The model under review builds one solid part; all positions refer to its coordinate system, in mm. A direction names the side the tool comes from. Give positions to 0.01 mm unless a question says otherwise; leave off trailing zeros. Loops run counter-clockwise (first coordinate to the right, second up) from the corner with the lowest first, then second, coordinate; pieces in that order, holes last. Notation, with made-up numbers: (14.25, 54) -> (46.25, 54) arc R13 cw to (46.25, 63) -> close; hole circle Ø8 at (-33, -8.5). An arc over 180 degrees is marked (long way). Write each question's results on one line, items separated by ' | '. Start each with the question number.
Q1. Mouldability with a two-part tool opening along X and no side actions: class faces 4 (the face through (-4.166, 1.398, 3.732)), 5 (the face through (11.68, 0.78, 3.7)), 6 (the face through (7, 1, 7.5)) as released by +X, released by -X, zero draft, split by the parting line, or undercut.
Q2. Insertion check: pin 1 Ø1.1 at (x, y) = (0, 0) entering from +Z; pin 2 Ø3 at (x, z) = (9.5, 6.5) entering from -Y; pin 3 Ø2.5 at (x, y) = (0, 1.5) entering from -Z; pin 4 Ø4.5 at (x, y) = (-1, 1.5) entering from +Z. Each pin has a flat end and moves straight along its axis. Give the tip position at first contact, or say it passes through.
Q3. We need section D-D (z = 0.5). Write out the cut boundary in (x, y).
Q4. We need section B-B (x = 0). Write out the cut boundary in (y, z).
Q5. We need section A-A (y = 0). Write out the cut boundary in (x, z), plus the area to 3 significant figures.
Q6. Wall thickness on L1, parallel to Y at x = 0, z = 4.05; L2, parallel to Z at x = -0.5, y = -1; L3, parallel to X at y = 0.75, z = 4: over which ranges is each line inside the solid? List them lowest first. Write a range as [from, to].
Q7. Machinability: for faces 1 (the face through (3, -3.761, 4)), 2 (the face through (-2, 1, 5)), 3 (the face through (-2, 1, 2.5)), which of the approach directions +Z, -Z, +X, -X, +Y, -Y give a long, thin tool a straight path to every point of the face, cutting with its end or side? Answer none if there is none.
Q8. We need section C-C (y = -1.75). Write out the cut boundary in (x, z).
from build123d import *

# Parameters (mm, degrees)
SKETCH1_R           = 0.8875
BOSS_EXTRUDE1_DEPTH = 7.5
SKETCH2_R           = 4.44
CUT_EXTRUDE1_DEPTH  = 2.5
CUT_EXTRUDE2_START  = -5
SKETCH2_2_R         = 4.44
CUT_EXTRUDE2_DEPTH  = 2.5


with BuildPart() as part:
    # Sketch1 → Boss-Extrude1 (new body)
    with BuildSketch(Plane.XY):
        with BuildLine():
            Line((-1.63988617, 5.119263092), (7.24011383, 5.119263092))
            ThreePointArc((7.24011383, 5.119263092), (11.68011383, 0.679263092), (7.24011383, -3.760736908))
            Line((7.24011383, -3.760736908), (-1.63988617, -3.760736908))
            ThreePointArc((-1.63988617, -3.760736908), (-6.07988617, 0.679263092), (-1.63988617, 5.119263092))
        make_face()
        Circle(SKETCH1_R, mode=Mode.SUBTRACT)
        with Locations((-3.27977234, 1.358526185)):
            Circle(SKETCH1_R, mode=Mode.SUBTRACT)
    extrude(amount=BOSS_EXTRUDE1_DEPTH)

    # Sketch2 → Cut-Extrude1 (cut)
    with BuildSketch(Plane(origin=(0, 0, 0), x_dir=(-1, 0, 0), z_dir=(0, 0, -1))):
        with Locations((1.63988617, 0.679263092)):
            Circle(SKETCH2_R)
    extrude(amount=-CUT_EXTRUDE1_DEPTH, mode=Mode.SUBTRACT)

    # Sketch2<2> → Cut-Extrude2 (cut)
    with BuildSketch(Plane(origin=(0, 0, 0), x_dir=(-1, 0, 0), z_dir=(0, 0, -1)).offset(CUT_EXTRUDE2_START)):
        with Locations((1.63988617, 0.679263092)):
            Circle(SKETCH2_2_R)
    extrude(amount=-CUT_EXTRUDE2_DEPTH, mode=Mode.SUBTRACT)


solid = part.part
Output:
1) face 4: undercut | face 5: released by +X | face 6: zero draft
2) pin 1: through | pin 2: y = -3.7 | pin 3: z = 2.5 | pin 4: z = 5
3) outline: (-1.64, -3.76) -> (7.24, -3.76) arc R4.44 ccw to (7.24, 5.12) -> (-1.64, 5.12) arc R4.44 cw to start
4) outline: (-3.76, 0) -> (-3.45, 0) -> (-3.45, 2.5) -> (-0.89, 2.5) -> (-0.89, 5) -> (-3.45, 5) -> (-3.45, 7.5) -> (-3.76, 7.5) -> close; (0.89, 2.5) -> (4.81, 2.5) -> (4.81, 0) -> (5.12, 0) -> (5.12, 7.5) -> (4.81, 7.5) -> (4.81, 5) -> (0.89, 5) -> close
5) outline: (-6.03, 2.5) -> (-0.89, 2.5) -> (-0.89, 5) -> (-6.03, 5) -> close; (0.89, 2.5) -> (2.75, 2.5) -> (2.75, 0) -> (11.63, 0) -> (11.63, 7.5) -> (2.75, 7.5) -> (2.75, 5) -> (0.89, 5) -> close | area: 84.1 mm2
6) L1: [-3.76, -0.89], [0.89, 5.12] | L2: [2.5, 5] | L3: [-6.08, -3.93], [-2.63, -0.47], [0.47, 11.68]
7) face 1: +Z, -Z, +X, -X, -Y | face 2: +Z, -X | face 3: -Z, -X
8) outline: (-5.36, 2.5) -> (2.08, 2.5) -> (2.08, 0) -> (10.96, 0) -> (10.96, 7.5) -> (2.08, 7.5) -> (2.08, 5) -> (-5.36, 5) -> close
